Input: dimensioned drawing with shaded views. Units: mm. Origin: part minimum x, y, z. A direction names the side the tool comes from. Coordinates: 2 decimals unless noted, no trailing zeros. Write each loop counter-clockwise with the first axis right and the second up, starting at its lowest first coordinate (ties: lowest second). Pieces come first, ordered by that corner, then holes. Notation, with made-up numbers: (15, 50.5) -> (59, 50.5) arc R15 cw to (59, 74.5) -> close; hole circle Ø5 at (46, 40). An arc over 180 degrees is marked (long way). One line per item, written item: value. Start each with the question number.
1. Section query B-B, the plane y = 126.5. Output: boundary loops of the cut face in (x, z).
2. Mould query, pull axis Z, two halves, no side actions, for the marked faces 4, 5 and 6. Classes: released by +Z, released by -Z, zero draft, split by the parting line, or undercut.
3. Section query A-A, the plane x = 317.5. Output: boundary loops of the cut face in (y, z) (1 decimal), and give its area (3 significant figures).
4. First-contact query: P1, Ø2, axis at x = 1216.5, y = 481, coming from the -Z side; P2, Ø12, axis at x = 829, y = 425, coming from the +Z side; P3, Ø2, axis at x = 542, z = 500, coming from the -Y side. Flat tips, straight axial feed; report the tip coordinate or a pass-through.
5. Section query D-D, the plane y = 532. Output: boundary loops of the cut face in (x, z).
6. Section query C-C, the plane z = 695.5. Output: boundary loops of the cut face in (x, y), and give its area (3 significant figures).
7. Access query for the marked faces 1, 2 and 3. Directions: +Z, -Z, +X, -X, +Y, -Y. A direction counts if a zero-diameter tool reaches every point of the face in a straight line with its end or side. Return the directions, or none.
8. Line query: line 1 (Z direction, x = 227, y = 290); line 2 (X direction, y = 87, z = 449); line 3 (Y direction, x = 1229.5, z = 528.5). Output: solid intervals per line, ascending.
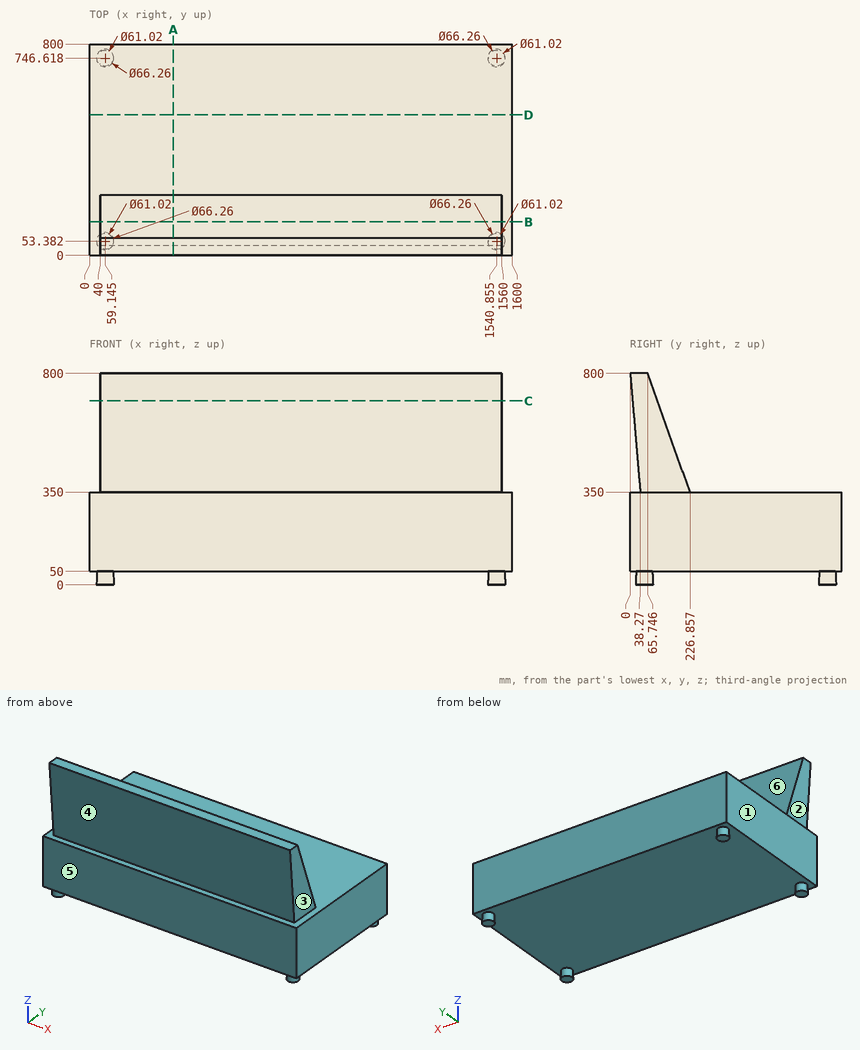
Computed values:
1. outline: (0, 50) -> (1600, 50) -> (1600, 350) -> (1560, 350) -> (1560, 630.31) -> (40, 630.31) -> (40, 350) -> (0, 350) -> close
2. face 4: undercut
2. face 5: zero draft
2. face 6: released by +Z
3. outline: (0, 50) -> (800, 50) -> (800, 350) -> (226.9, 350) -> (65.7, 800) -> (0, 800) -> (38.3, 350) -> (0, 350) -> close
3. area: 297,000 mm²
4. P1: stops at z = 50
4. P2: stops at z = 350
4. P3: stops at y = 25.43
5. outline: (0, 50) -> (1600, 50) -> (1600, 350) -> (0, 350) -> close
6. outline: (40, 8.89) -> (1560, 8.89) -> (1560, 103.16) -> (40, 103.16) -> close
6. area: 143,000 mm²
7. face 1: +Z, -Z, -X, +Y, -Y
7. face 2: +Z, -X, +Y, -Y
7. face 3: +Z, +X, +Y, -Y
8. line 1: z = 50 to 350
8. line 2: x = 40 to 1560
8. line 3: y = 23.09 to 162.95
